Build history of the part. All positions in model axes, mm. Face numbers are marked on the shaded views. A direction names the side the tool comes from. Round coordinates to 2 decimals unless told otherwise and drop trailing zeros. Order: outer loops, then holes, each group sorted by start corner. A loop starts at its lowest first (then second) coordinate and runs counter-clockwise, first axis right, second up. Notation, with made-up numbers: (68, -2) - (122, -2) arc R20 ccw to (122, 8) - close; hole circle Ø11 at (82.5, -3.75). An arc over 180 degrees is marked (long way). One line per question, with ' | ' between items. Start each with the question number.
from build123d import *

# Parameters (mm, degrees)
CUT_EXTRUDE_START   = -11
SKETCH_2_W          = 16
SKETCH_2_H          = 5
CUT_EXTRUDE_4_DEPTH = 29


with BuildPart() as part:
    # 草图1 → 旋转1 (revolve)
    with BuildSketch(Plane(origin=(0, 0, 0), x_dir=(0, 0, -1), z_dir=(1, 0, 0)), mode=Mode.PRIVATE) as revolve_1_sk:
        Polygon((40, 0), (40, 6), (0, 6), (0, 36.5), (-3, 36.5), (-3, 39.5), (-100, 39.5), (-100, 0), align=None)
    revolve(revolve_1_sk.sketch.rotate(Axis((0, 0, 105), (0, 0, -1)), 90), axis=Axis((0, 0, 105), (0, 0, -1)))

    # 草图2 → 切除-拉伸4 (cut)
    with BuildSketch(Plane.XY.offset(CUT_EXTRUDE_START)):
        with Locations((0, 7.5)):
            Rectangle(SKETCH_2_W, SKETCH_2_H)
    extrude(amount=-CUT_EXTRUDE_4_DEPTH, mode=Mode.SUBTRACT)


solid = part.part
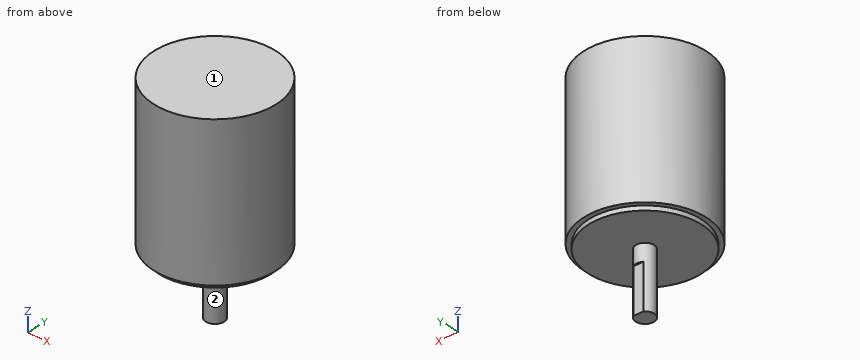
Item 1: 3-axis set-ups, long thin cutter, end or side, ignore diameter. For the marked faces 1 and 2: which of +Z, -Z, +X, -X, +Y, -Y reach the whole face in a straight line?
Item 2: Slice it at B-B (x = 0). Write the cut outline in (y, z).
Item 3: Pin check, flat tips, straight feed: pin 1 (3 mm diameter, centred on x = 17, z = 54.5, fed in from -Y); pin 2 (6 mm diameter, centred on y = 12.5, z = 18.5, fed in from -X); pin 3 (3 mm diameter, centred on x = -24, z = 10, fed in from -Y). Stop position of each tip, or through.
Item 4: Slice it at A-A (y = -18). Write the cut outline in (x, z), plus the area to 3 significant figures.
Item 5: Slice it at C-C (z = -28). Write the cut outline in (x, y), plus the area to 3 significant figures.
Item 6: Slice it at D-D (y = 0). Write the cut outline in (x, z).
Item 7: Wall check: line 1 along Z through (x, y) = (5, -6.5); line 2 along X through (y, z) = (-1.5, 68); line 3 along Z through (x, y) = (22, -29.5). Give the ranges that are in metal, low to high. Write a range as [from, to].
A:
1) face 1: +Z, +X, -X, +Y, -Y | face 2: -Z
2) outline: (-39.5, 3) - (-36.5, 3) - (-36.5, 0) - (-6, 0) - (-6, -40) - (5, -40) - (5, -11) - (6, -11) - (6, 0) - (36.5, 0) - (36.5, 3) - (39.5, 3) - (39.5, 100) - (-39.5, 100) - close
3) pin 1: y = -36.33 | pin 2: x = -38.34 | pin 3: y = -32.47
4) outline: (-35.16, 3) - (-31.75, 3) - (-31.75, 0) - (31.75, 0) - (31.75, 3) - (35.16, 3) - (35.16, 100) - (-35.16, 100) - close | area: 7,010 mm^2
5) outline: (-3.32, 5) arc R6 ccw (long way) to (3.32, 5) - close | area: 109 mm^2
6) outline: (-39.5, 3) - (-36.5, 3) - (-36.5, 0) - (-6, 0) - (-6, -40) - (6, -40) - (6, 0) - (36.5, 0) - (36.5, 3) - (39.5, 3) - (39.5, 100) - (-39.5, 100) - close
7) line 1: [0, 100] | line 2: [-39.47, 39.47] | line 3: [3, 100]
